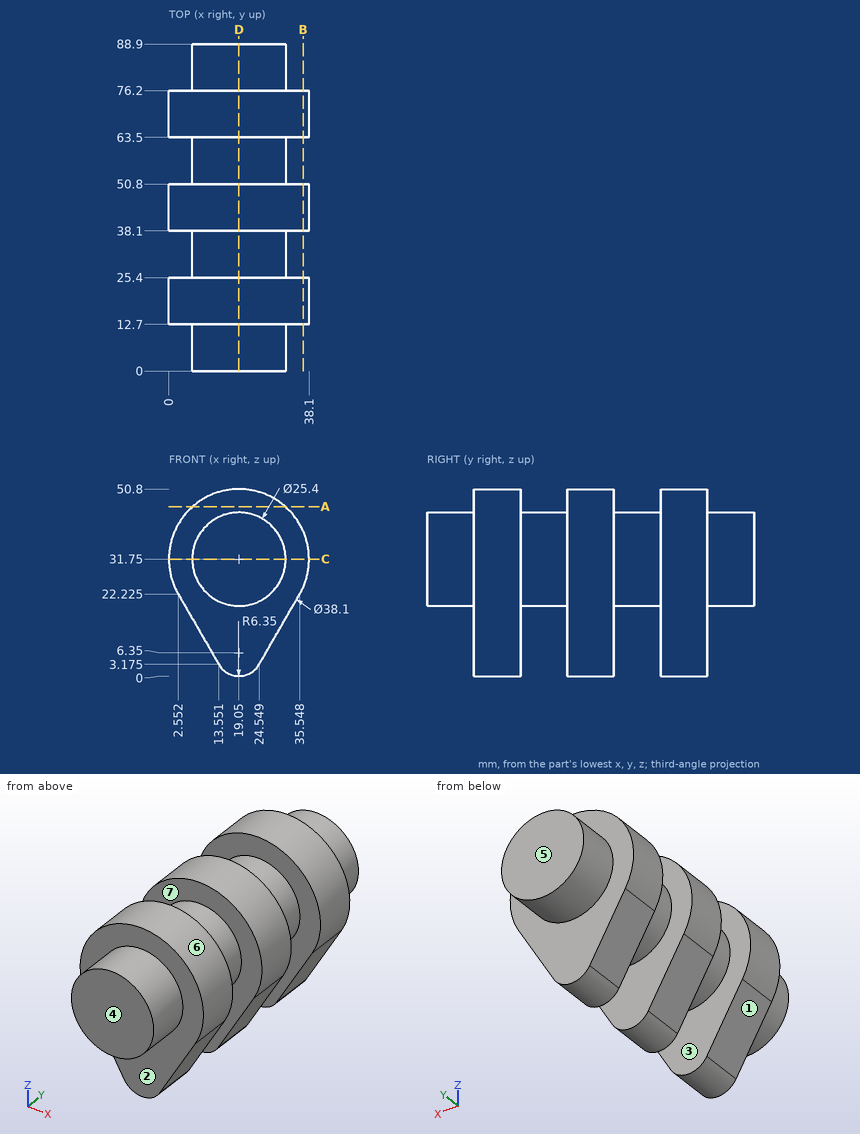
Answer from the drawing. Dimensions are ordinates in mm from the lowest x, y and z of the part. A direction names the side the tool comes from. Give positions to 0.01 mm unless a question says otherwise; leave off trailing zeros. Order: outer loops, then holes, each group sorted by start corner. A loop starts at its lowest first (then second) coordinate and runs counter-clockwise, first axis right, second up. Notation, with made-up numbers: (3.25, -25) -> (8.25, -25) arc R13 cw to (8.25, -1) -> close; hole circle Ø5 at (10.25, 74.5). An arc over 180 degrees is marked (long way). Answer as a JSON object with one key per item and string values. Group by question number.
1. Flat-ended cylindrical pins translate along their axes: pin 1 Ø10 at (x, z) = (31.5, 10) entering from +Y; pin 2 Ø12 at (x, y) = (8.5, 14) entering from +Z; pin 3 Ø2 at (x, z) = (29.5, 16) entering from -Y. Find the tip coordinate at first contact, or state that the pin passes through.
2. Section A-A on z = 46 is taken. Determine the outline of the cut face in (x, y).
3. Section D-D on x = 19.05 is taken. Determine the outline of the cut face in (y, z), plus the area to 3 significant figures.
4. Consider line 1 along Y through (x, z) = (35, 34.5); line 2 along Z through (x, y) = (6.5, 44) (1 decimal); line 3 along Z through (x, y) = (30.5, 9.5) (1 decimal). Determine where each line is inside the solid, lowest interval first. Write a range as [from, to].
5. Section C-C on z = 31.75 is taken. Determine the outline of the cut face in (x, y), plus the area to 3 significant figures.
6. The mould has two halves that part along Y. Classify the marked faces 4, 5, 6 and 7: released by +Y, released by -Y, zero draft, split by the parting line, or undercut.
7. Section B-B on x = 36.5 is taken. Determine the outline of the cut face in (y, z), plus the area to 3 significant figures.
8. A tool of negligible diameter and unlimited length cuts with its end or side. For the marked faces 1, 2 and 3, from which of +Z, -Z, +X, -X, +Y, -Y can it reach the whole face along a straight path? Write none if from no direction.
Result sheet:
{
 "1": {"pin 1": "stops at y = 76.2", "pin 2": "stops at z = 50.25", "pin 3": "stops at y = 12.7"},
 "2": {"outline": "(6.41, 12.7) -> (31.69, 12.7) -> (31.69, 25.4) -> (6.41, 25.4) -> close; (6.41, 38.1) -> (31.69, 38.1) -> (31.69, 50.8) -> (6.41, 50.8) -> close; (6.41, 63.5) -> (31.69, 63.5) -> (31.69, 76.2) -> (6.41, 76.2) -> close"},
 "3": {"outline": "(0, 19.05) -> (12.7, 19.05) -> (12.7, 0) -> (25.4, 0) -> (25.4, 19.05) -> (38.1, 19.05) -> (38.1, 0) -> (50.8, 0) -> (50.8, 19.05) -> (63.5, 19.05) -> (63.5, 0) -> (76.2, 0) -> (76.2, 19.05) -> (88.9, 19.05) -> (88.9, 44.45) -> (76.2, 44.45) -> (76.2, 50.8) -> (63.5, 50.8) -> (63.5, 44.45) -> (50.8, 44.45) -> (50.8, 50.8) -> (38.1, 50.8) -> (38.1, 44.45) -> (25.4, 44.45) -> (25.4, 50.8) -> (12.7, 50.8) -> (12.7, 44.45) -> (0, 44.45) -> close", "area": "3,230 mm^2"},
 "4": {"line 1": "y = [12.7, 25.4], [38.1, 50.8], [63.5, 76.2]", "line 2": "z = [15.4, 46.1]", "line 3": "z = [26.3, 37.2]"},
 "5": {"outline": "(0, 12.7) -> (6.35, 12.7) -> (6.35, 0) -> (31.75, 0) -> (31.75, 12.7) -> (38.1, 12.7) -> (38.1, 25.4) -> (31.75, 25.4) -> (31.75, 38.1) -> (38.1, 38.1) -> (38.1, 50.8) -> (31.75, 50.8) -> (31.75, 63.5) -> (38.1, 63.5) -> (38.1, 76.2) -> (31.75, 76.2) -> (31.75, 88.9) -> (6.35, 88.9) -> (6.35, 76.2) -> (0, 76.2) -> (0, 63.5) -> (6.35, 63.5) -> (6.35, 50.8) -> (0, 50.8) -> (0, 38.1) -> (6.35, 38.1) -> (6.35, 25.4) -> (0, 25.4) -> close", "area": "2,740 mm^2"},
 "6": {"face 4": "released by -Y", "face 5": "released by +Y", "face 6": "zero draft", "face 7": "undercut"},
 "7": {"outline": "(12.7, 24.11) -> (25.4, 24.11) -> (25.4, 39.39) -> (12.7, 39.39) -> close; (38.1, 24.11) -> (50.8, 24.11) -> (50.8, 39.39) -> (38.1, 39.39) -> close; (63.5, 24.11) -> (76.2, 24.11) -> (76.2, 39.39) -> (63.5, 39.39) -> close", "area": "582 mm^2"},
 "8": {"face 1": "-Z, -X, +Y, -Y", "face 2": "-Y", "face 3": "none"}
}
